Work out the finished part from the listing and answer in its coordinate system (mm). A direction names the side the tool comes from. Give positions to 0.01 mm unless a question says otherwise; leave off trailing zeros. Order: outer loops, then holes, each group sorted by start corner. A loop starts at its lowest first (then second) coordinate and runs counter-clockwise, first axis right, second up. Notation, with made-up numbers: M -37.75,55 L -17.75,55 A13 ccw -17.75,70 Z; hole C -26,8.5 d2. An arc over 180 degrees is marked long. One line per item, written item: value.
from build123d import *

# Parameters (mm, degrees)
SKETCH_1_R      = 3
EXTRUDE_1_DEPTH = 6
SKETCH_2_R      = 3
EXTRUDE_2_DEPTH = 12
EXTRUDE_3_DEPTH = 3
EXTRUDE_4_DEPTH = 12
EXTRUDE_5_DEPTH = 12


with BuildPart() as part:
    # 스케치1 → 보스-돌출1 (new, symmetric)
    with BuildSketch(Plane(origin=(0, 0, 0), x_dir=(0, 0, -1), z_dir=(1, 0, 0))):
        with BuildLine():
            Line((-12, 12), (12, 12))
            Line((12, 12), (7.101042921, -2.413542921))
            ThreePointArc((7.101042921, -2.413542921), (0, -7.5), (-7.101042921, -2.413542921))
            Line((-7.101042921, -2.413542921), (-12, 12))
        make_face()
        Circle(SKETCH_1_R, mode=Mode.SUBTRACT)
    extrude(amount=EXTRUDE_1_DEPTH, both=True)

    # 스케치2 → 보스-돌출2 (add)
    with BuildSketch(Plane(origin=(0, 12, 0), x_dir=(1, 0, 0), z_dir=(0, 1, 0))):
        with BuildLine():
            Line((-12, -9), (12, -9))
            Line((12, -9), (7.319153043, -22.637070166))
            ThreePointArc((7.319153043, -22.637070166), (0.403262311, -28.489150787), (-7.101042921, -23.413542921))
            Line((-7.101042921, -23.413542921), (-12, -9))
        make_face()
        with Locations(Location((0, -21, 0), (0, 0, 270))):
            Circle(SKETCH_2_R, mode=Mode.SUBTRACT)
    extrude(amount=EXTRUDE_2_DEPTH)

    # 스케치3 → 보스-돌출3 (add)
    with BuildSketch(Plane(origin=(0, 0, 9), x_dir=(-1, 0, 0), z_dir=(0, 0, -1))):
        Polygon((-12, 12), (-6, 12), (6, 12), (12, 12), (12, 24), (-12, 24), align=None)
    extrude(amount=EXTRUDE_3_DEPTH)

    # 스케치4 → 보스-돌출4 (add)
    with BuildSketch(Plane(origin=(0, 0, 6), x_dir=(-1, 0, 0), z_dir=(0, 0, -1))):
        Polygon((-9, 12), (-6, 9), (-6, 12), (6, 12), (6, 9), (9, 12), (12, 12), (12, 24), (-12, 24), (-12, 12), align=None)
    extrude(amount=EXTRUDE_4_DEPTH)

    # 스케치5 → 보스-돌출5 (add)
    with BuildSketch(Plane(origin=(0, 12, 0), x_dir=(1, 0, 0), z_dir=(0, 1, 0))):
        Polygon((-12, 6), (12, 6), (9, 12), (-9, 12), align=None)
    extrude(amount=EXTRUDE_5_DEPTH)


solid = part.part
(1) Given P1, Ø6, axis at x = -4.5, y = 7, coming from the +Z side; P2, Ø10, axis at x = -6, z = 18, coming from the -Y side; P3, Ø5, axis at x = -3.5, z = 8, coming from the -Y side; P4, Ø3.5, axis at x = 0, z = 21, coming from the +Y side, each flat-ended and moving along its own axis, determine where each tip first touches the part or whether it passes through.
Findings:
P1: stops at z = 11.32
P2: stops at y = 12
P3: stops at y = -5.1
P4: passes through
(2) Section B-B, the plane y = 20 is taken. Give the vertices of the cut face in (x, z).
Findings:
outline: M -12,-6 L -9,-12 L 9,-12 L 12,-6 L 12,9 L 7.32,22.64 A7.5 ccw -7.1,23.41 L -12,9 Z; hole C 0,21 d6
(3) Section A-A, the plane x = 0 is taken. Give the vertices of the cut face in (y, z), then the cut area to 3 significant figures.
Findings:
outline: M -2.41,-7.1 L 12,-12 L 24,-12 L 24,18 L 12,18 L 12,12 L -2.41,7.1 A7.5 ccw Z; M 12,24 L 24,24 L 24,28.5 L 12,28.5 Z; hole C 0,0 d6
area: 714 mm^2
(4) Which of the six approach directions +Z, -Z, +X, -X, +Y, -Y give full straight-line access (tool end or side, diameter ignored) to faces 1 (the flat face through (-7, 11, -6)), 2 (the flat face through (-7, 11, 6)), 3 (the flat face through (8, 11, 0))?
Findings:
face 1: -Z, -X, -Y
face 2: +Z, -X, -Y
face 3: +Z, -Z, +X, -Y
(5) Determine the mould class of faces 4 (the flat face through (-7, 10, 0)), 5 (the cylindrical face through (0, 18, 18)), 6 (the cylindrical face through (0, 0, 3)), 7 (the flat face through (7, 11, -6)) for opening direction Z: pulls with the +Z half, pulls with the -Z half, needs draft (parallel to the pull), parting line crosses it, or undercut.
Findings:
face 4: needs draft
face 5: undercut
face 6: undercut
face 7: pulls with the -Z half
(6) Section C-C, the plane z = 0 is taken. Give the vertices of the cut face in (x, y).
Findings:
outline: M -12,12 L -9,12 L -6,9 L -6,3 L 6,3 L 6,9 L 9,12 L 12,12 L 12,24 L -12,24 Z; M -6,-7.5 L 6,-7.5 L 6,-3 L -6,-3 Z
(7) Find the intervals of material crossed by probe 1 along Y at (x, z) = (-2.5, 0); probe 2 along Y at (x, z) = (7.75, 12); probe 3 along X at (y, z) = (6.5, 3.5), in increasing order. Write a range as from..to.
Findings:
probe 1: y = -7.5..-3, 3..24
probe 2: y = 12..24
probe 3: x = -6..6
(8) Section D-D, the plane z = 6.5 is taken. Give the vertices of the cut face in (x, y), then the cut area to 3 significant figures.
Findings:
outline: M -12,12 L -6,12 L -6,-3.74 L 6,-3.74 L 6,12 L 12,12 L 12,24 L -12,24 Z
area: 477 mm^2
